Can you work these out from the model? Positions are in its coordinate system, mm. Face numbers are marked on the shaded views. A direction names the side the tool comes from. Give positions to 0.01 mm unless a question says otherwise; leave off trailing zeros. Order: outer loops, then holes, each group sorted by start corner. A loop starts at its lowest first (then second) coordinate and runs counter-clockwise, first axis right, second up. Notation, with made-up numbers: (7, 43.5) - (58, 43.5) arc R20 cw to (58, 59.5) - close; hole circle Ø1 at (-22.5, 57.25). An arc over 180 degrees is marked (long way). Answer as CSV lines item,"result".
Autodesk Inventor part; units mm, degrees
ref_plane "YZ Plane" through (0, 0, 0) normal (1, 0, 0) x (0, 1, 0)
ref_plane "XZ Plane" through (0, 0, 0) normal (0, 1, 0) x (-1, 0, 0)
ref_plane "XY Plane" through (0, 0, 0) normal (0, 0, 1) x (1, 0, 0)
sketch "Sketch1" plane through (0, 0, 0) normal (0, 1, 0) x (-1, 0, 0)
  line L0 (0, 0) -> (0, -20)
  line L1 (0, -20) -> (15, -20)
  line L2 (15, -20) -> (15, -27)
  line L3 (15, -27) -> (0, -27)
  line L4 (0, 0) -> (15, 0)
  line L5 (15, 0) -> (15, 7)
  line L6 (15, 7) -> (0, 7)
  line L7 (-4, -20) -> (0, -20)
  circle A0 centre (-4, -5) radius 1.6
  circle A1 centre (-4, -15) radius 1.6
  line L8 (0, 7) -> (-12, 7)
  line L9 (-12, 7) -> (-12, -27)
  line L10 (-12, -27) -> (0, -27)
  line L11 (0, -20) -> (-12, -20)
  line L12 (-12, 0) -> (-12, 7)
  line L13 (0, 0) -> (-4, 0)
  line L14 (-4, 0) -> (-12, 0)
  line L15 (15, 0) -> (-12, 0)
  line L16 (0, 7) -> (0, 0)
  line L17 (0, -20) -> (0, -27)
  line L18 (-4, -8) -> (-12, -8)
  line L19 (-4, -8) -> (0, -8)
  line L20 (-4, -2) -> (-12, -2)
  line L21 (-4, -2) -> (0, -2)
  line L22 (-4, -18) -> (0, -18)
  line L23 (-4, -18) -> (-12, -18)
  line L24 (-4, -12) -> (-12, -12)
  line L25 (-4, -12) -> (0, -12)
  dimension "d0" = 20
  dimension "d1" = 15
  dimension "d2" = 7
  dimension "d4" = 7
  dimension "d5" = 4
extrude "Extrusion1" add sketch "Sketch1" along normal blind 20 contours L16 L6 L5 L4 | L13 L14 L9 L8 L16 | L17 L10 L9 L11 L7 | L1 L2 L3 L17
extrude "Extrusion2" add sketch "Sketch1" along normal blind 9 contours L0 L21 L20 L9 L14 L13 | L0 L19 L18 L9 L20 L21 | L0 L25 L24 L9 L18 L19 | L0 L22 L23 L9 L24 L25 | L0 L7 L11 L9 L23 L22
extrude "Extrusion3" add sketch "Sketch1" against normal blind 15 contours L0 L21 L20 L9 L14 L13 | L13 L14 L9 L8 L16 | L0 L25 L24 L9 L18 L19 | L0 L7 L11 L9 L23 L22 | L17 L10 L9 L11 L7
extrude "Extrusion4" add sketch "Sketch1" against normal blind 10 contours L0 L19 L18 L9 L20 L21 | L0 L22 L23 L9 L24 L25
sketch "Sketch2" plane through (-15, 20, 7) normal (0, 0, 1) x (1, 0, 0)
  line L0 (15, -20) -> (15, 0)
  line L1 (0, 0) -> (27, 0)
  line L2 (15, 0) -> (27, 0)
  line L3 (27, 0) -> (27, -35)
  line L4 (27, -35) -> (15, -35)
  line L5 (15, -35) -> (15, -20)
extrude "Extrusion5" add sketch "Sketch2" along normal blind 4
sketch "Sketch3" plane through (12, 20, -27) normal (0, 0, -1) x (-1, 0, 0)
  line L0 (0, -35) -> (12, -35)
  line L1 (12, -35) -> (12, 0)
  line L2 (12, 0) -> (0, 0)
  line L3 (27, 0) -> (0, 0)
  line L4 (0, 0) -> (0, -35)
  line L5 (0, -35) -> (0, 0)
  point P0 (12, -20)
extrude "Extrusion6" add sketch "Sketch3" along normal blind 4
sketch "Sketch4" plane through (12, 9, -20) normal (1, 0, 0) x (0, 0, -1)
  line L0 (-31, -24) -> (-18, -24)
  line L1 (-18, -24) -> (-31, -24)
  line L2 (-24.5, -24) -> (-24.5, -16)
  line L3 (-2, -24) -> (11, -24)
  line L4 (4.5, -24) -> (4.5, -16)
  circle A0 centre (-24.5, -16) radius 2.65
  circle A1 centre (4.5, -16) radius 2.65
  point P0 (-20, -9)
  dimension "d27" = 8
  dimension "d28" = 8
  dimension "d29" = 5.3
  dimension "d30" = 5.3
extrude "Extrusion7" cut sketch "Sketch4" against normal blind 13
properties part number "servo_clip_holder1"
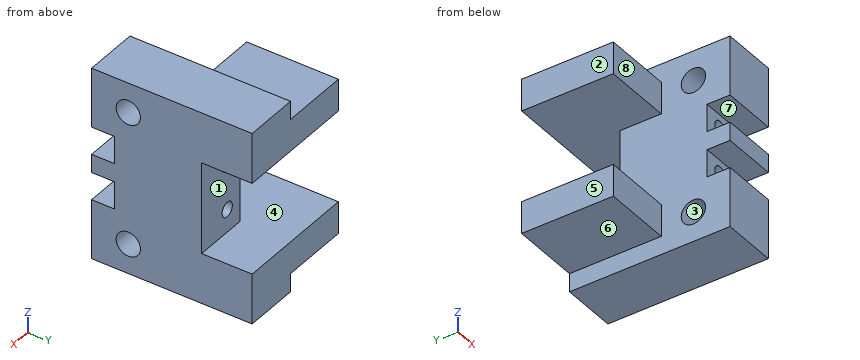
1) Which directions (+Z, -Z, +X, -X, +Y, -Y) give clear straight access to the entire face, cutting with the end or side of a thin tool? Please do the marked faces 4, 5, 6, 7 and 8.
Answer block:
face 4,"-X, +Y"
face 5,"+Z, -Z, -X, +Y, -Y"
face 6,"-Z, -X, +Y, -Y"
face 7,"+X, -X, -Y"
face 8,"+Z, -Z, -X, -Y"
2) I need wall thicknesses on line 1 along Z through (x, y) = (4, -2.25); line 2 along Y through (x, z) = (8, -24.5); line 3 along Z through (x, y) = (-1.5, 17). Which ranges of each line are inside material? Lowest first, please. Write a range as [from, to].
Answer block:
line 1,"[-31, -16.6], [-13.4, -6.6], [-3.4, 11]"
line 2,"[-15, -9.65], [-4.35, 20]"
line 3,"[-27, -20], [0, 7]"
3) I want a section at C-C on x = 4. Write out the boundary of the cut face in (y, z), plus the area to 3 significant figures.
Answer block:
outline,"(-15, -31) - (20, -31) - (20, -20) - (9, -20) - (9, -16.6) - (-10, -16.6) - (-10, -18) - (-15, -18) - close; (-15, -12) - (-10, -12) - (-10, -13.4) - (9, -13.4) - (9, -6.6) - (-10, -6.6) - (-10, -8) - (-15, -8) - close; (-15, -2) - (-10, -2) - (-10, -3.4) - (9, -3.4) - (9, 0) - (20, 0) - (20, 11) - (-15, 11) - close; hole circle Ø5.3 at (-7, -24.5); hole circle Ø5.3 at (-7, 4.5)"
area,"1,020 mm2"
4) I want a section at A-A on y = -7. Write out the boundary of the cut face in (x, z), plus the area to 3 significant figures.
Answer block:
outline,"(0, -31) - (12, -31) - (12, -27.15) - (0, -27.15) - close; (0, -21.85) - (12, -21.85) - (12, 1.85) - (0, 1.85) - close; (0, 7.15) - (12, 7.15) - (12, 11) - (0, 11) - close; hole circle Ø3.2 at (4, -15); hole circle Ø3.2 at (4, -5)"
area,"361 mm2"
5) I want a section at B-B on x = -1.25. Write out the boundary of the cut face in (y, z).
Answer block:
outline,"(0, -27) - (20, -27) - (20, -20) - (0, -20) - close; (0, 0) - (20, 0) - (20, 7) - (0, 7) - close"
6) I want a section at D-D on y = 15. Write out the boundary of the cut face in (x, z).
Answer block:
outline,"(-15, -27) - (0, -27) - (0, -31) - (12, -31) - (12, -20) - (-15, -20) - close; (-15, 0) - (12, 0) - (12, 11) - (0, 11) - (0, 7) - (-15, 7) - close"
7) I'm going to push flat-ended pins straight in: P1, Ø8, axis at y = 13.5, z = -17, coming from the +X side; P2, Ø1.5, axis at x = -2.5, z = -2.5, coming from the +Y side; P3, Ø4.5, axis at x = -10.5, y = 6.5, coming from the +Z side; P4, Ø3, axis at x = 4.5, z = -4.5, coming from the -Y side. Where does each tip first touch, or does it pass through?
Answer block:
P1,"x = 12"
P2,"through"
P3,"z = 7"
P4,"y = -10"
8) If we mould it in two halves opening along Y, with no side actions, what happens to the marked faces 1, 2 and 3? For each: +Y half, -Y half, draft (parallel to the pull), parting line (faces both ways), or undercut.
Answer block:
face 1,"+Y half"
face 2,"draft"
face 3,"undercut"
